from build123d import *

# Parameters (mm, degrees)
BOSS_EXTRUDE1_DEPTH = 251
CUT_EXTRUDE1_REACH  = 253.194
SKETCH3_R           = 2.5


with BuildPart() as part:
    # Sketch2 → Boss-Extrude1 (new body)
    with BuildSketch(Plane(origin=(0, 0, 0), x_dir=(0, 0, -1), z_dir=(1, 0, 0))):
        Polygon((-4, 4.25), (-4, -3.25), (4, -3.25), (4, 4.25), (5, 4.25), (5, -4.25), (-5, -4.25), (-5, 4.25), align=None)
    extrude(amount=BOSS_EXTRUDE1_DEPTH)

    # Sketch3 → Cut-Extrude1 (cut, up to next)
    with BuildSketch(Plane.XZ.offset(4.25), mode=Mode.PRIVATE) as cut_extrude1_sk1:
        with Locations(Location((19, 0, 0), (0, 0, 270))):
            Circle(SKETCH3_R)
    cut_extrude1_tool1 = extrude(cut_extrude1_sk1.sketch, amount=-CUT_EXTRUDE1_REACH, mode=Mode.PRIVATE) & part.part
    # Sketch3 → Cut-Extrude1 (cut, up to next)
    with BuildSketch(Plane.XZ.offset(4.25), mode=Mode.PRIVATE) as cut_extrude1_sk2:
        with Locations(Location((27.5, 0, 0), (0, 0, 270))):
            Circle(SKETCH3_R)
    cut_extrude1_tool2 = extrude(cut_extrude1_sk2.sketch, amount=-CUT_EXTRUDE1_REACH, mode=Mode.PRIVATE) & part.part
    # Sketch3 → Cut-Extrude1 (cut, up to next)
    with BuildSketch(Plane.XZ.offset(4.25), mode=Mode.PRIVATE) as cut_extrude1_sk3:
        with Locations(Location((36, 0, 0), (0, 0, 270))):
            Circle(SKETCH3_R)
    cut_extrude1_tool3 = extrude(cut_extrude1_sk3.sketch, amount=-CUT_EXTRUDE1_REACH, mode=Mode.PRIVATE) & part.part
    # Sketch3 → Cut-Extrude1 (cut, up to next)
    with BuildSketch(Plane.XZ.offset(4.25), mode=Mode.PRIVATE) as cut_extrude1_sk4:
        with Locations(Location((115, 0, 0), (0, 0, 270))):
            Circle(SKETCH3_R)
    cut_extrude1_tool4 = extrude(cut_extrude1_sk4.sketch, amount=-CUT_EXTRUDE1_REACH, mode=Mode.PRIVATE) & part.part
    # Sketch3 → Cut-Extrude1 (cut, up to next)
    with BuildSketch(Plane.XZ.offset(4.25), mode=Mode.PRIVATE) as cut_extrude1_sk5:
        with Locations(Location((123.5, 0, 0), (0, 0, 270))):
            Circle(SKETCH3_R)
    cut_extrude1_tool5 = extrude(cut_extrude1_sk5.sketch, amount=-CUT_EXTRUDE1_REACH, mode=Mode.PRIVATE) & part.part
    # Sketch3 → Cut-Extrude1 (cut, up to next)
    with BuildSketch(Plane.XZ.offset(4.25), mode=Mode.PRIVATE) as cut_extrude1_sk6:
        with Locations(Location((132, 0, 0), (0, 0, 270))):
            Circle(SKETCH3_R)
    cut_extrude1_tool6 = extrude(cut_extrude1_sk6.sketch, amount=-CUT_EXTRUDE1_REACH, mode=Mode.PRIVATE) & part.part
    # Sketch3 → Cut-Extrude1 (cut, up to next)
    with BuildSketch(Plane.XZ.offset(4.25), mode=Mode.PRIVATE) as cut_extrude1_sk7:
        with Locations(Location((232, 0, 0), (0, 0, 270))):
            Circle(SKETCH3_R)
    cut_extrude1_tool7 = extrude(cut_extrude1_sk7.sketch, amount=-CUT_EXTRUDE1_REACH, mode=Mode.PRIVATE) & part.part
    # Sketch3 → Cut-Extrude1 (cut, up to next)
    with BuildSketch(Plane.XZ.offset(4.25), mode=Mode.PRIVATE) as cut_extrude1_sk8:
        with Locations(Location((223.5, 0, 0), (0, 0, 270))):
            Circle(SKETCH3_R)
    cut_extrude1_tool8 = extrude(cut_extrude1_sk8.sketch, amount=-CUT_EXTRUDE1_REACH, mode=Mode.PRIVATE) & part.part
    # Sketch3 → Cut-Extrude1 (cut, up to next)
    with BuildSketch(Plane.XZ.offset(4.25), mode=Mode.PRIVATE) as cut_extrude1_sk9:
        with Locations(Location((215, 0, 0), (0, 0, 270))):
            Circle(SKETCH3_R)
    cut_extrude1_tool9 = extrude(cut_extrude1_sk9.sketch, amount=-CUT_EXTRUDE1_REACH, mode=Mode.PRIVATE) & part.part
    add(cut_extrude1_tool1.solids().sort_by_distance((19, -4.25, 0))[0], mode=Mode.SUBTRACT)
    add(cut_extrude1_tool2.solids().sort_by_distance((27.5, -4.25, 0))[0], mode=Mode.SUBTRACT)
    add(cut_extrude1_tool3.solids().sort_by_distance((36, -4.25, 0))[0], mode=Mode.SUBTRACT)
    add(cut_extrude1_tool4.solids().sort_by_distance((115, -4.25, 0))[0], mode=Mode.SUBTRACT)
    add(cut_extrude1_tool5.solids().sort_by_distance((123.5, -4.25, 0))[0], mode=Mode.SUBTRACT)
    add(cut_extrude1_tool6.solids().sort_by_distance((132, -4.25, 0))[0], mode=Mode.SUBTRACT)
    add(cut_extrude1_tool7.solids().sort_by_distance((232, -4.25, 0))[0], mode=Mode.SUBTRACT)
    add(cut_extrude1_tool8.solids().sort_by_distance((223.5, -4.25, 0))[0], mode=Mode.SUBTRACT)
    add(cut_extrude1_tool9.solids().sort_by_distance((215, -4.25, 0))[0], mode=Mode.SUBTRACT)


solid = part.part
Here's how the part is built. I have some questions about the finished solid (model axes, mm). A direction names the side the tool comes from. Give positions to 0.01 mm unless a question says otherwise; leave off trailing zeros. Order: outer loops, then holes, each group sorted by start corner. A loop starts at its lowest first (then second) coordinate and runs counter-clockwise, first axis right, second up. Notation, with made-up numbers: (-2, 67) -> (11, 67) arc R20 cw to (11, 104) -> close; hole circle Ø11 at (70.5, -0.75). An arc over 180 degrees is marked (long way). One line per item, written item: value. Start each with the question number.
1. Will this pin go through, and if not, where does the flat tip stop? pin 1 Ø2.5 at (x, z) = (150, 0) entering from +Y.
2. I need wall thicknesses on probe 1 along Z at (x, y) = (36.5, 3.75); probe 2 along Y at (x, z) = (196, -1.5). Which ranges of each line are inside material? Lowest first, please. Write a range as from..to.
3. Imagine slicing it at C-C, the plane x = 154. List the corners of the cut face in (y, z) for me.
4. Imagine slicing it at A-A, the plane x = 123.5. List the corners of the cut face in (y, z) for me, plus the area to 3 significant figures.
5. We'd pull the mould along Z, two halves only. Please class faces 3 (the face through (124, 0, -5)), 4 (the face through (251, -3.44, -0.02)), 5 (the face through (33.56, -3.76, 0.54)): released by +Z, released by -Z, zero draft, split by the parting line, or undercut.
6. Imagine slicing it at B-B, the plane y = -1. List the corners of the cut face in (x, z) for me, plus the area to 3 significant figures.
7. For faces 1 (the face through (124, 0, 5)), 2 (the face through (124, -3.25, 3)), which set-ups out of +Z, -Z, +X, -X, +Y, -Y let a thin tool reach every point of the face, with its end or its side?
8. Imagine slicing it at D-D, the plane z = 0. Count the separate pieces of the cut face and the enclosed holes in it, plus the area to 3 significant figures.
Values follow:
1. pin 1: stops at y = -3.25
2. probe 1: z = -5..-4, 4..5
2. probe 2: y = -4.25..-3.25
3. outline: (-4.25, -5) -> (4.25, -5) -> (4.25, -4) -> (-3.25, -4) -> (-3.25, 4) -> (4.25, 4) -> (4.25, 5) -> (-4.25, 5) -> close
4. outline: (-4.25, -5) -> (4.25, -5) -> (4.25, -4) -> (-3.25, -4) -> (-3.25, -2.5) -> (-4.25, -2.5) -> close; (-4.25, 2.5) -> (-3.25, 2.5) -> (-3.25, 4) -> (4.25, 4) -> (4.25, 5) -> (-4.25, 5) -> close
4. area: 20.0 mm2
5. face 3: released by -Z
5. face 4: zero draft
5. face 5: undercut
6. outline: (0, -5) -> (251, -5) -> (251, -4) -> (0, -4) -> close; (0, 4) -> (251, 4) -> (251, 5) -> (0, 5) -> close
6. area: 502 mm2
7. face 1: +Z, +X, -X, +Y, -Y
7. face 2: +X, -X, +Y
8. separate pieces: 10
8. enclosed holes: 0
8. area: 206 mm2
